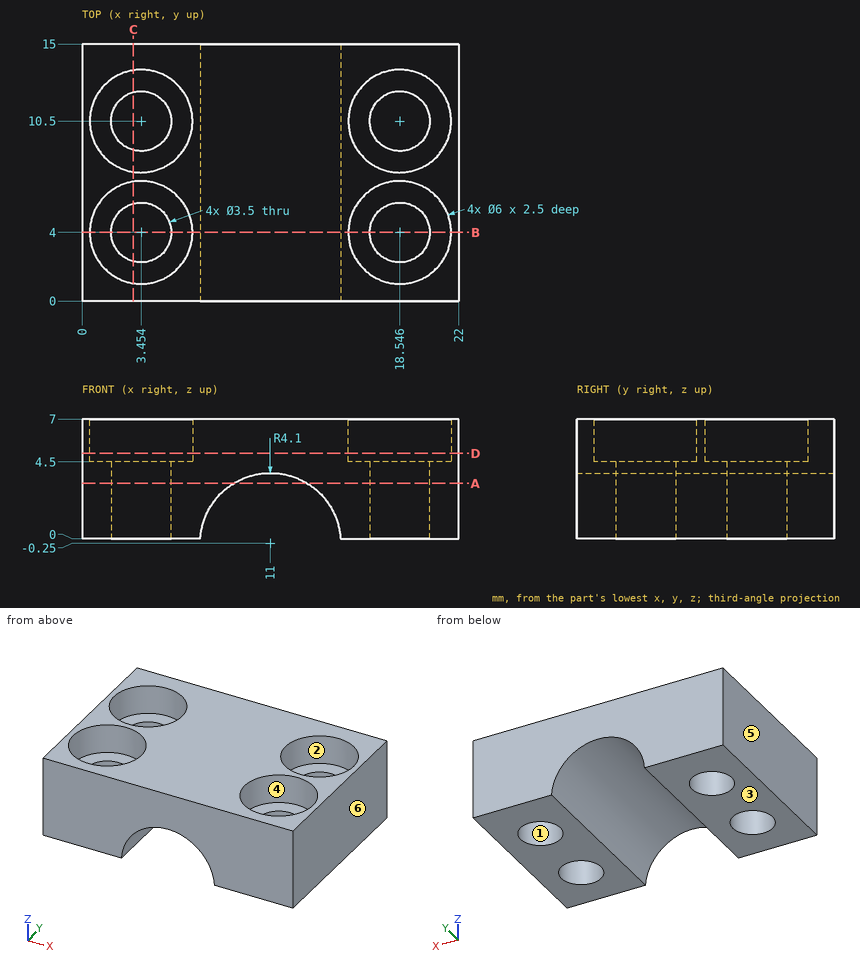
Study the drawing (mm; zero at the part's minimum x, y, z) and answer. A direction names the side the tool comes from. Round coordinates to 2 decimals unless told otherwise and drop trailing zeros. Loops run counter-clockwise (first coordinate to the right, second up) from the corner with the lowest first, then second, coordinate; pieces in that order, holes last. Notation, with made-up numbers: (49, -30) - (93, -30) arc R34 ccw to (93, 1) - close; hole circle Ø11 at (3, 27). An arc over 180 degrees is marked (long way). Use one line per item in the form item = value. Start each with the question number.
1. Given pin 1 Ø3 at (x, y) = (3.45, 10.5) entering from -Z; pin 2 Ø1.8 at (x, y) = (19, 11.5) entering from +Z; pin 3 Ø1.5 at (x, y) = (11.5, 2) entering from -Z (1 decimal); pin 4 Ø1.5 at (x, y) = (14, 7.5) entering from -Z, each flat-ended and moving along its own axis, determine where each tip first touches the part or whether it passes through.
2. The part is cut by section D-D on z = 5. Determine the outline of the cut face in (x, y), then the cut area to 3 significant figures.
3. A tool of negligible diameter and unlimited length cuts with its end or side. For the marked faces 1 and 2, from which of +Z, -Z, +X, -X, +Y, -Y can it reach the whole face along a straight path? Write none if from no direction.
4. Consider line 1 (Y direction, x = 18.5, z = 6); line 2 (X direction, y = 3.25, z = 4.25) (1 decimal); line 3 (Y direction, x = 4.5, z = 3). Determine where each line is inside the solid, lowest interval first. Write a range as [from, to].
5. The part is cut by section B-B on y = 4. Determine the outline of the cut face in (x, z).
6. The part is cut by section C-C on x = 3. Determine the outline of the cut face in (y, z).
7. For a pull along X with two mould halves and no side action, classify the marked faces 3, 4, 5 and 6 as pulls with the +X half, pulls with the -X half, needs draft (parallel to the pull), parting line crosses it, or undercut.
8. The part is cut by section A-A on z = 3.25. Determine the outline of the cut face in (x, y).
Geometry check:
q1.pin_1 = through
q1.pin_2 = 4.5
q1.pin_3 = 3.7
q1.pin_4 = 1.41
q2.outline = (0, 0) - (22, 0) - (22, 15) - (0, 15) - close; hole circle Ø6 at (3.45, 4); hole circle Ø6 at (3.45, 10.5); hole circle Ø6 at (18.55, 4); hole circle Ø6 at (18.55, 10.5)
q2.area = 217 mm^2
q3.face_1 = +Z, -Z
q3.face_2 = +Z
q4.line_1 = [0, 1], [7, 7.5], [13.5, 15]
q4.line_2 = [0, 1.9], [5, 17], [20.1, 22]
q4.line_3 = [0, 2.6], [5.4, 9.1], [11.9, 15]
q5.outline = (0, 0) - (1.7, 0) - (1.7, 4.5) - (0.45, 4.5) - (0.45, 7) - (0, 7) - close; (5.2, 0) - (6.91, 0) arc R4.1 cw to (15.09, 0) - (16.8, 0) - (16.8, 4.5) - (15.55, 4.5) - (15.55, 7) - (6.45, 7) - (6.45, 4.5) - (5.2, 4.5) - close; (20.3, 0) - (22, 0) - (22, 7) - (21.55, 7) - (21.55, 4.5) - (20.3, 4.5) - close
q6.outline = (0, 0) - (2.31, 0) - (2.31, 4.5) - (1.03, 4.5) - (1.03, 7) - (0, 7) - close; (5.69, 0) - (8.81, 0) - (8.81, 4.5) - (7.53, 4.5) - (7.53, 7) - (6.97, 7) - (6.97, 4.5) - (5.69, 4.5) - close; (12.19, 0) - (15, 0) - (15, 7) - (13.47, 7) - (13.47, 4.5) - (12.19, 4.5) - close
q7.face_3 = needs draft
q7.face_4 = undercut
q7.face_5 = pulls with the -X half
q7.face_6 = pulls with the +X half
q8.outline = (0, 0) - (8.86, 0) - (8.86, 15) - (0, 15) - close; (13.14, 0) - (22, 0) - (22, 15) - (13.14, 15) - close; hole circle Ø3.5 at (3.45, 4); hole circle Ø3.5 at (3.45, 10.5); hole circle Ø3.5 at (18.55, 4); hole circle Ø3.5 at (18.55, 10.5)
